```python
from build123d import *

# Parameters (mm, degrees)
HOLE_WIZARD_1_D     = 5.917
HOLE_WIZARD_1_DEPTH = 14.8
HOLE_WIZARD_1_TIP   = 1.777646141
CHAMFER_1_SIZE      = 0.5


with BuildPart() as part:
    # Эскиз1 → Повернуть1 (revolve)
    with BuildSketch(Plane(origin=(0, 0, 0), x_dir=(0, 0, -1), z_dir=(1, 0, 0))):
        Polygon((-4, 42.7), (-4, 34.7), (-2.1, 33.603034489), (-2.1, 0), (-11.15, 0), (-11.15, 1), (-6.099727925, 1), (-5.968494929, 2.5), (-11.15, 2.5), (-11.15, 3.5), (-5.881006266, 3.5), (-5.749773271, 5), (-11.15, 5), (-11.15, 6), (-5.662284607, 6), (-5.531051612, 7.5), (-11.15, 7.5), (-11.15, 8.5), (-5.443562948, 8.5), (-5.312329953, 10), (-11.15, 10), (-11.15, 11), (-5.224841289, 11), (-5.093608294, 12.5), (-11.15, 12.5), (-11.15, 13.5), (-5.006119631, 13.5), (-4.874886635, 15), (-11.15, 15), (-11.15, 16), (-4.787397972, 16), (-4.656164976, 17.5), (-11.15, 17.5), (-11.15, 18.5), (-4.568676313, 18.5), (-4.437443318, 20), (-11.15, 20), (-11.15, 21), (-4.349954654, 21), (-4.218721659, 22.5), (-11.15, 22.5), (-11.15, 23.5), (-4.131232995, 23.5), (-4, 25), (-11.15, 25), (-11.15, 26), (-4, 26), (-4, 27.5), (-8, 27.5), (-8, 28.5), (-4, 28.5), (-4, 30), (-8, 30), (-8, 33), (-6, 33), (-6, 39), (-8, 39), (-8, 42.7), align=None)
    revolve(axis=Axis((0, 0, 0), (0, 1, 0)))

    # Отверстие1
    with Locations(Plane.XZ):
        with Locations((0, 0)):
            Hole(HOLE_WIZARD_1_D / 2, depth=HOLE_WIZARD_1_DEPTH)
            with Locations((0, 0, -(HOLE_WIZARD_1_DEPTH + HOLE_WIZARD_1_TIP / 2))):  # 118° drill point
                Cone(0, HOLE_WIZARD_1_D / 2, HOLE_WIZARD_1_TIP, mode=Mode.SUBTRACT)

    # Фаска1
    chamfer_1_edges = [part.edges().sort_by_distance(p)[0] for p in [
        (2.9585, 0, 0),
    ]]
    chamfer(chamfer_1_edges, length=CHAMFER_1_SIZE)


solid = part.part
```
Geometry check sheet. Reference: the model listing, model coordinates, mm. A direction names the side the tool comes from. Give positions to 0.01 mm unless a question says otherwise; leave off trailing zeros. Write each loop counter-clockwise with the first axis right and the second up, starting at its lowest first coordinate (ties: lowest second). Pieces come first, ordered by that corner, then holes. Notation, with made-up numbers: (-5, 5.25) -> (38, 5.25) arc R7 ccw to (38, 15.25) -> close; hole circle Ø2 at (16, 12). An arc over 180 degrees is marked (long way). One line per question, with ' | ' between items.
Item 1: Sectioned sample at A-A, the plane y = 35.5. Record the boundary of the cut face in (x, z), plus the area to 3 significant figures.
Determined:
outline: circle Ø12 at (0, 0); hole circle Ø8 at (0, 0) | area: 62.8 mm^2
Item 2: Sectioned sample at B-B, the plane x = -8.75. State how many separate pieces and enclosed holes the cut face has, plus the area to 3 significant figures.
Determined:
separate pieces: 11 | enclosed holes: 0 | area: 152 mm^2
Item 3: Scan lines: line 1 along X through (y, z) = (10.25, 0); line 2 along X through (y, z) = (40.5, 0); line 3 along X through (y, z) = (30.5, 5.5). Record each from-to range of solid material in increasing order.
Determined:
line 1: -11.15 to -2.96, 2.96 to 11.15 | line 2: -8 to -4, 4 to 8 | line 3: -5.81 to 5.81
Item 4: Sectioned sample at D-D, the plane y = 20.5. Record the boundary of the cut face in (x, z), plus the area to 3 significant figures.
Determined:
outline: circle Ø22.3 at (0, 0); hole circle Ø4.2 at (0, 0) | area: 377 mm^2
Item 5: Depth check by flat-ended pin: pin 1 (1 mm diameter, centred on x = -6.5, y = 18.5, fed in from +Z); pin 2 (8 mm diameter, centred on x = 4, y = 33.5, fed in from +Z); pin 3 (4 mm diameter, centred on y = 30, z = -4, fed in from +X). Enter the tip coordinate at first touch or a pass-through.
Determined:
pin 1: z = 9.4 | pin 2: z = 8 | pin 3: x = 7.75
Item 6: Draft check along Y on faces 4 (the cylindrical face through (-3.905, 38.644, -0.867)), 5 (the flat face through (-5, 8.5, -3)), 6 (the flat face through (3, 0, 3)). Enter one of: released by +Y, released by -Y, zero draft, split by the parting line, or undercut.
Determined:
face 4: zero draft | face 5: undercut | face 6: released by -Y
Item 7: Access from +Z, -Z, +X, -X, +Y, -Y to the whole of each face (thin tool, end or side, straight path). Record for faces 1 (the cylindrical face through (-7.81, 40.88, -1.73)), 2 (the flat face through (-5, 12.5, -2)), 3 (the cylindrical face through (0.631, 24.331, 2.003)).
Determined:
face 1: +Y | face 2: none | face 3: +Y, -Y
